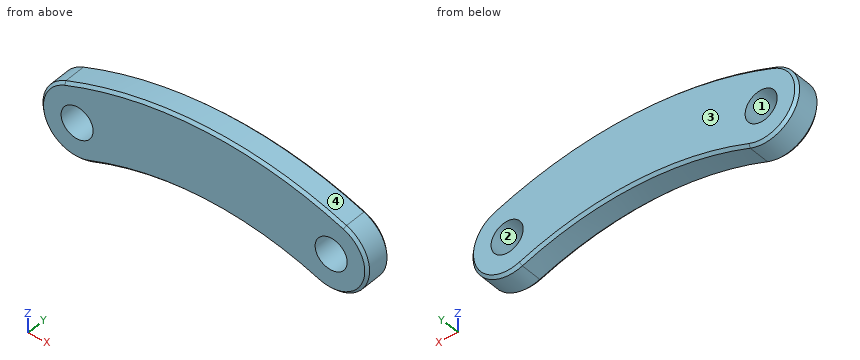
from build123d import *

# Parameters (mm, degrees)
SKETCH_1_R      = 3
EXTRUDE_1_DEPTH = 5
CHAMFER_1_SIZE  = 0.5


with BuildPart() as part:
    # 草图1 → 凸台-拉伸1 (new body)
    with BuildSketch(Plane(origin=(0, 0, 0), x_dir=(1, 0, 0), z_dir=(0, 1, 0))):
        with BuildLine():
            ThreePointArc((45.140425532, 6.339597261), (53.935193412, 2.470895471), (50.082208589, -6.330769347))
            ThreePointArc((50.082208589, -6.330769347), (23.8, -11.299093911), (-2.482208589, -6.330769347))
            ThreePointArc((-2.482208589, -6.330769347), (-6.335193412, 2.470895471), (2.459574468, 6.339597261))
            ThreePointArc((2.459574468, 6.339597261), (23.8, 2.344926441), (45.140425532, 6.339597261))
        make_face()
        Circle(SKETCH_1_R, mode=Mode.SUBTRACT)
        with Locations((47.6, 0)):
            Circle(SKETCH_1_R, mode=Mode.SUBTRACT)
    extrude(amount=EXTRUDE_1_DEPTH)

    # 倒角1
    chamfer_1_edges = [part.edges().sort_by_distance(p)[0] for p in [
        (23.8, 5, 11.299093911),
        (53.935193412, 5, -2.470895471),
        (23.8, 5, -2.344926441),
        (53.935193412, 0, -2.470895471),
        (23.8, 0, 11.299093911),
        (-6.335193412, 0, -2.470895471),
        (23.8, 0, -2.344926441),
        (-6.335193412, 5, -2.470895471),
    ]]
    chamfer(chamfer_1_edges, length=CHAMFER_1_SIZE)


solid = part.part
The listing builds one solid part. Answer for the finished solid, in the listing's coordinates (mm). Face numbers are marked on the shaded views. Round coordinates to 2 decimals unless told otherwise and drop trailing zeros. Write each loop counter-clockwise with the first axis right and the second up, starting at its lowest first coordinate (ties: lowest second). Pieces come first, ordered by that corner, then holes. Notation, with made-up numbers: (76, 56) - (93, 56) arc R38 ccw to (93, 94) - close; hole circle Ø7 at (30, 55.25). An arc over 180 degrees is marked (long way). Use a Markdown table: item, result. Add a question column.
1. For a pull along X with two mould halves and no side action, classify the marked faces 1, 2, 3 and 4 as +X half, -X half, draft (parallel to the pull), parting line (faces both ways), or undercut.
2. Consider line 1 (X direction, y = 2.25, z = 0); line 2 (Z direction, x = 0, y = 3.8); line 3 (Z direction, x = 46, y = 2.6). Determine where each line is inside the solid, lowest interval first.
3. The part is cut by section A-A (z = 0). Write down the section's boundary in (x, y).
4. The part is cut by section B-B (y = 2.75). Write down the section's boundary in (x, z).
Reported:
| question | item | result |
|---|---|---|
| 1 | face 1 | undercut |
| 1 | face 2 | undercut |
| 1 | face 3 | draft |
| 1 | face 4 | parting line |
| 2 | line 1 | -6.8 to -3, 3 to 44.6, 50.6 to 54.4 |
| 2 | line 2 | -6.8 to -3, 3 to 7.25 |
| 2 | line 3 | -6.61 to -2.54, 2.54 to 7.79 |
| 3 | outline | (-6.8, 0.5) - (-6.3, 0) - (-3, 0) - (-3, 5) - (-6.3, 5) - (-6.8, 4.5) - close; (3, 0) - (44.6, 0) - (44.6, 5) - (3, 5) - close; (50.6, 0) - (53.9, 0) - (54.4, 0.5) - (54.4, 4.5) - (53.9, 5) - (50.6, 5) - close |
| 4 | outline | (-2.48, 6.33) arc R6.8 ccw to (2.46, -6.34) arc R59 cw to (45.14, -6.34) arc R6.8 ccw to (50.08, 6.33) arc R72 ccw to start; hole circle Ø6 at (0, 0); hole circle Ø6 at (47.6, 0) |
